Geometry check sheet. Reference: the model listing, model coordinates, mm. A direction names the side the tool comes from. Coordinates: 2 decimals unless noted, no trailing zeros. Write each loop counter-clockwise with the first axis right and the second up, starting at its lowest first coordinate (ties: lowest second). Pieces come first, ordered by that corner, then holes. Notation, with made-up numbers: (9.5, -21.5) -> (43.5, -21.5) arc R29 cw to (43.5, 3.5) -> close; hole circle Ø2 at (45, -28). An arc over 180 degrees is marked (long way). Use a Markdown table: item, result.
```python
from build123d import *

# Parameters (mm, degrees)
SKETCH1_W               = 17.78
SKETCH1_H               = 2.54
BOSS_EXTRUDE1_DEPTH     = 11.43
SKETCH2_W               = 17.78
SKETCH2_H               = 2.54
BOSS_EXTRUDE2_DEPTH     = 15.24
SKETCH16_W              = 3.81
SKETCH16_H              = 2.54
BOSS_EXTRUDE10_DEPTH    = 7.62
BOSS_EXTRUDE11_REACH    = 36.757
SKETCH17_W              = 5.08
SKETCH17_H              = 2.54
MIRROR3_COPY_1_SKETCH_W = 3.81
MIRROR3_COPY_1_SKETCH_H = 2.54
MIRROR3_COPY_1_DEPTH    = 7.62
MIRROR3_COPY_2_REACH    = 36.757
MIRROR3_COPY_2_SKETCH_W = 5.08
MIRROR3_COPY_2_SKETCH_H = 2.54
FILLET1_R               = 2.54
SKETCH18_W              = 5.0165
SKETCH18_H              = 17.78
BOSS_EXTRUDE12_DEPTH    = 5.0165
SKETCH19_W              = 17.78
SKETCH19_H              = 2.4765
BOSS_EXTRUDE13_DEPTH    = 5.0165


with BuildPart() as part:
    # Sketch1 → Boss-Extrude1 (new body)
    with BuildSketch(Plane(origin=(0, 0, 0), x_dir=(0, 0, -1), z_dir=(1, 0, 0))):
        with Locations((0, 1.27)):
            Rectangle(SKETCH1_W, SKETCH1_H)
    extrude(amount=BOSS_EXTRUDE1_DEPTH)

    # Sketch2 → Boss-Extrude2 (add)
    with BuildSketch(Plane.ZY):
        with Locations((0, 1.27)):
            Rectangle(SKETCH2_W, SKETCH2_H)
    extrude(amount=BOSS_EXTRUDE2_DEPTH)

    # Mirror1: part across plane


with BuildPart() as part_1:
    add(part.part)
    add(part.part.mirror(Plane.ZY.offset(15.24)))

    # Sketch16 → Boss-Extrude10 (add)
    with BuildSketch(Plane.XY.offset(8.89)):
        with Locations((-17.145, 1.27)):
            Rectangle(SKETCH16_W, SKETCH16_H)
        with Locations((-40.005, 1.27)):
            Rectangle(SKETCH16_W, SKETCH16_H)
    boss_extrude10 = extrude(amount=BOSS_EXTRUDE10_DEPTH)

    # Sketch17 → Boss-Extrude11 (add, up to next)
    with BuildSketch(Plane.ZY.offset(19.05), mode=Mode.PRIVATE) as boss_extrude11_sk1:
        with Locations((13.97, 1.27)):
            Rectangle(SKETCH17_W, SKETCH17_H)
    boss_extrude11_tool1 = extrude(boss_extrude11_sk1.sketch, amount=BOSS_EXTRUDE11_REACH, mode=Mode.PRIVATE) - part_1.part
    boss_extrude11 = boss_extrude11_tool1.solids().sort_by_distance((-19.05, 1.27, 13.97))[0]
    add(boss_extrude11)

    # Mirror2: Boss-Extrude10, Boss-Extrude11 across plane
    add(boss_extrude10.mirror(Plane.ZY.offset(15.24)))
    add(boss_extrude11.mirror(Plane.ZY.offset(15.24)))

    # Mirror3: Boss-Extrude10, Boss-Extrude11 across plane
    add(boss_extrude10.mirror(Plane.XY))
    add(boss_extrude11.mirror(Plane.XY))

    # Mirror3 copy 1 sketch → Mirror3 copy 1 (add)
    with BuildSketch(Plane(origin=(-30.48, 0, -8.89), x_dir=(-1, 0, 0), z_dir=(0, 0, -1))):
        with Locations((-17.145, 1.27)):
            Rectangle(MIRROR3_COPY_1_SKETCH_W, MIRROR3_COPY_1_SKETCH_H)
        with Locations((-40.005, 1.27)):
            Rectangle(MIRROR3_COPY_1_SKETCH_W, MIRROR3_COPY_1_SKETCH_H)
    extrude(amount=MIRROR3_COPY_1_DEPTH)

    # Mirror3 copy 2 sketch → Mirror3 copy 2 (add, up to next)
    with BuildSketch(Plane(origin=(-11.43, 0, 0), x_dir=(0, 0, -1), z_dir=(1, 0, 0)), mode=Mode.PRIVATE) as mirror3_copy_2_sk1:
        with Locations((13.97, 1.27)):
            Rectangle(MIRROR3_COPY_2_SKETCH_W, MIRROR3_COPY_2_SKETCH_H)
    mirror3_copy_2_tool1 = extrude(mirror3_copy_2_sk1.sketch, amount=MIRROR3_COPY_2_REACH, mode=Mode.PRIVATE) - part_1.part
    add(mirror3_copy_2_tool1.solids().sort_by_distance((-11.43, 1.27, -13.97))[0])

    # Fillet1
    fillet1_edges = [part_1.edges().sort_by_distance(p)[0] for p in [
        (-41.91, 1.27, -16.51),
        (11.43, 1.27, -16.51),
        (-41.91, 1.27, 16.51),
        (11.43, 1.27, 16.51),
    ]]
    fillet(fillet1_edges, radius=FILLET1_R)

    # Sketch18 → Boss-Extrude12 (add)
    with BuildSketch(Plane.XZ):
        with Locations((-12.73175, 0)):
            Rectangle(SKETCH18_W, SKETCH18_H)
    boss_extrude12 = extrude(amount=BOSS_EXTRUDE12_DEPTH)

    # Sketch19 → Boss-Extrude13 (add)
    with BuildSketch(Plane(origin=(-10.2235, 0, 0), x_dir=(0, 0, -1), z_dir=(1, 0, 0))):
        with Locations((0, -3.77825)):
            Rectangle(SKETCH19_W, SKETCH19_H)
    boss_extrude13 = extrude(amount=BOSS_EXTRUDE13_DEPTH)

    # Mirror4: Boss-Extrude12, Boss-Extrude13 across plane
    add(boss_extrude12.mirror(Plane.ZY.offset(15.24)))
    add(boss_extrude13.mirror(Plane.ZY.offset(15.24)))


solid = part_1.part
```
Item 1: Section check B-B on z = -10. Record the boundary of the cut face in (x, y), then the cut area to 3 significant figures.
Answer block:
| item | result |
|---|---|
| outline | (-41.91, 0) -> (-38.1, 0) -> (-38.1, 2.54) -> (-41.91, 2.54) -> close; (-19.05, 0) -> (-11.43, 0) -> (-11.43, 2.54) -> (-19.05, 2.54) -> close; (7.62, 0) -> (11.43, 0) -> (11.43, 2.54) -> (7.62, 2.54) -> close |
| area | 38.7 mm^2 |
Item 2: Tool access check on faces 4 (the flat face through (-20.257, -1, 0)), 5 (the flat face through (-5.207, -4, 0)), 6 (the flat face through (-11.43, 1, 10)). Record the directions out of +Z, -Z, +X, -X, +Y, -Y that give a thin tool (end or side, any length) a straight path to the whole face; none if there is none.
Answer block:
| item | result |
|---|---|
| face 4 | +Z, -Z, -X |
| face 5 | +Z, -Z, +X, -Y |
| face 6 | +Y, -Y |
Item 3: Section check D-D on y = 1. Record the boundary of the cut face in (x, z).
Answer block:
| item | result |
|---|---|
| outline | (-41.91, -13.97) arc R2.54 ccw to (-39.37, -16.51) -> (8.89, -16.51) arc R2.54 ccw to (11.43, -13.97) -> (11.43, 13.97) arc R2.54 ccw to (8.89, 16.51) -> (-39.37, 16.51) arc R2.54 ccw to (-41.91, 13.97) -> close; hole (-38.1, -11.43) -> (-19.05, -11.43) -> (-19.05, -8.89) -> (-38.1, -8.89) -> close; hole (-38.1, 8.89) -> (-19.05, 8.89) -> (-19.05, 11.43) -> (-38.1, 11.43) -> close; hole (-11.43, -11.43) -> (7.62, -11.43) -> (7.62, -8.89) -> (-11.43, -8.89) -> close; hole (-11.43, 8.89) -> (7.62, 8.89) -> (7.62, 11.43) -> (-11.43, 11.43) -> close |
Item 4: Thickness scan on L1, parallel to Z at x = -33.5, y = 2.25; L2, parallel to Y at x = -7, z = -6; L3, parallel to Y at x = 8, z = 14. Record the ranges inside material, lowest first. Write a range as [from, to].
Answer block:
| item | result |
|---|---|
| L1 | z = [-16.51, -11.43], [-8.89, 8.89], [11.43, 16.51] |
| L2 | y = [-5.02, -2.54], [0, 2.54] |
| L3 | y = [0, 2.54] |
Item 5: Section check A-A on x = -32. Record the boundary of the cut face in (y, z).
Answer block:
| item | result |
|---|---|
| outline | (0, -16.51) -> (2.54, -16.51) -> (2.54, -11.43) -> (0, -11.43) -> close; (0, -8.89) -> (2.54, -8.89) -> (2.54, 8.89) -> (0, 8.89) -> close; (0, 11.43) -> (2.54, 11.43) -> (2.54, 16.51) -> (0, 16.51) -> close |
Item 6: Mould release check, pull along X, two halves, no side actions. Record for faces 1 (the flat face through (-8, -2.54, 0)), 2 (the cylindrical face through (-41.146, 1.288, 15.786)), 3 (the flat face through (-2, 1, 11.43)): +X half, -X half, draft (parallel to the pull), parting line (faces both ways), or undercut.
Answer block:
| item | result |
|---|---|
| face 1 | draft |
| face 2 | -X half |
| face 3 | undercut |
Item 7: Section check C-C on x = -21. Record the boundary of the cut face in (y, z).
Answer block:
| item | result |
|---|---|
| outline | (-5.02, -8.89) -> (-2.54, -8.89) -> (-2.54, 8.89) -> (-5.02, 8.89) -> close; (0, -16.51) -> (2.54, -16.51) -> (2.54, -11.43) -> (0, -11.43) -> close; (0, -8.89) -> (2.54, -8.89) -> (2.54, 8.89) -> (0, 8.89) -> close; (0, 11.43) -> (2.54, 11.43) -> (2.54, 16.51) -> (0, 16.51) -> close |
Item 8: Depth check by flat-ended pin: P1, Ø0.8, axis at y = -1, z = -3, coming from the -X side; P2, Ø1.5, axis at x = -26.5, z = -2, coming from the -Y side; P3, Ø0.7, axis at y = -3.5, z = -3.5, coming from the +X side. Enter the tip coordinate at first touch or a pass-through.
Answer block:
| item | result |
|---|---|
| P1 | stops at x = -20.26 |
| P2 | stops at y = 0 |
| P3 | stops at x = -5.21 |
